Design review of the part shown in the three views and the two pictorial views. Dimensions are in mm from the part's minimum x, y and z. A direction names the side the tool comes from. Round coordinates to 2 decimals unless told otherwise and drop trailing zeros. Loops run counter-clockwise (first coordinate to the right, second up) from the corner with the lowest first, then second, coordinate; pieces in that order, holes last. Notation, with made-up numbers: (37.5, 36.5) -> (90.5, 36.5) arc R19 cw to (90.5, 51.5) -> close; hole circle Ø8 at (1.25, 59.25). An arc over 180 degrees is marked (long way). Write each question's results on one line, items separated by ' | '. Start each with the question number.
Item 1: For L1, parallel to X at y = 16, z = 3.85; L2, parallel to Y at x = 53.5, z = 1.1; L3, parallel to Y at x = 62.5, z = 4.6 (1 decimal), list the stretches that pass through material, from the lowest coordinate up. Write a range as from..to.
Item 2: We need section A-A (z = 3.9). Give the number of separate pieces and of enclosed holes in the cut face, and give its area (3 significant figures).
Item 3: We need section C-C (x = 53.5). Give the boundary of the cut face in (y, z).
Item 4: Mouldability with a two-part tool opening along Y and no side actions: class the marked faces 1, 2, 3 and 4 as pulls with the +Y half, pulls with the -Y half, needs draft (parallel to the pull), parting line crosses it, or undercut.
Item 5: Tool access review of the marked faces 5 and 6: name each direction out of +Z, -Z, +X, -X, +Y, -Y from which nothing blocks a thin tool from reaching the whole face with its end or side.
Item 6: We need section B-B (y = 18.5). Give the boundary of the cut face in (x, z).
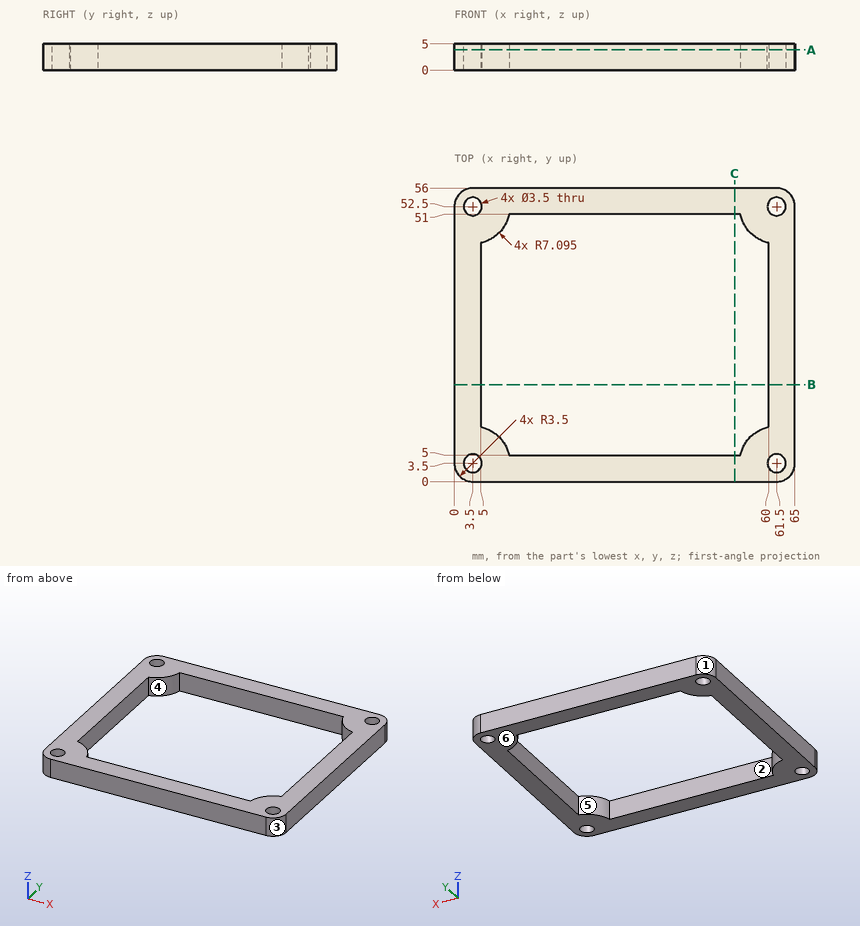
Here are the results:
1) L1: x = 0..5, 60..65 | L2: y = 0..5, 51..56 | L3: y = 0.1..2.1, 4.9..51.1, 53.9..55.9
2) separate pieces: 1 | enclosed holes: 5 | area: 1,140 mm2
3) outline: (0, 0) -> (5, 0) -> (5, 5) -> (0, 5) -> close; (51, 0) -> (56, 0) -> (56, 5) -> (51, 5) -> close
4) face 1: pulls with the +Y half | face 2: undercut | face 3: pulls with the -Y half | face 4: undercut
5) face 5: +Z, -Z | face 6: -Z, +X, -X, +Y, -Y
6) outline: (0, 0) -> (5, 0) -> (5, 5) -> (0, 5) -> close; (60, 0) -> (65, 0) -> (65, 5) -> (60, 5) -> close
